Could you check a few things on this model? Use its own coordinates, in mm. Face numbers are marked on the shaded views. A direction names the side the tool comes from. Coordinates: 2 decimals unless noted, no trailing zeros. Order: outer loops, then holes, each group sorted by start corner. A loop starts at its lowest first (then second) coordinate and runs counter-clockwise, first axis right, second up. Notation, with made-up numbers: (86.5, 77) - (134.5, 77) arc R30 ccw to (134.5, 110) - close; hole circle Ø8 at (-4.5, 28). An arc over 180 degrees is marked (long way). Answer as CSV lines item,"result". Start each with the question number.
1. For the marked faces 4, 5, 6 and 7, which set-ups out of +Z, -Z, +X, -X, +Y, -Y let a thin tool reach every point of the face, with its end or its side?
2. I want a section at D-D, the plane z = -18. List the corners of the cut face in (x, y) for me, and give its area (3 significant figures).
3. I want a section at B-B, the plane y = 3. List the corners of the cut face in (x, z) for me, and give its area (3 significant figures).
4. I want a section at A-A, the plane z = 0. List the corners of the cut face in (x, y) for me.
5. I need wall thicknesses on probe 1 along X at (y, z) = (3.65, 0); probe 2 along Z at (x, y) = (15.75, 3); probe 3 along Z at (x, y) = (-1.75, 2.25). Which ranges of each line are inside material? Lowest first, please.
6. For pin 1 (1.2 mm diameter, centred on x = 8, y = 8.5, fed in from +Z); pin 2 (6 mm diameter, centred on y = 7.5, z = -29.5, fed in from +X); pin 3 (0.9 mm diameter, centred on x = 7.5, y = 2.5, fed in from +Z); pin 4 (3 mm diameter, centred on x = 0, z = 0, fed in from +Y), each with a flat end and sliding along its axis, tell me the tip position at first contact or that it passes through.
7. I want a section at C-C, the plane x = 15. List the corners of the cut face in (y, z) for me, and give its area (3 significant figures).
8. Thinking about a two-plate mould opening in X: for the marked faces 1, 2 and 3, which applies, released by +X, released by -X, zero draft, split by the parting line, or undercut?
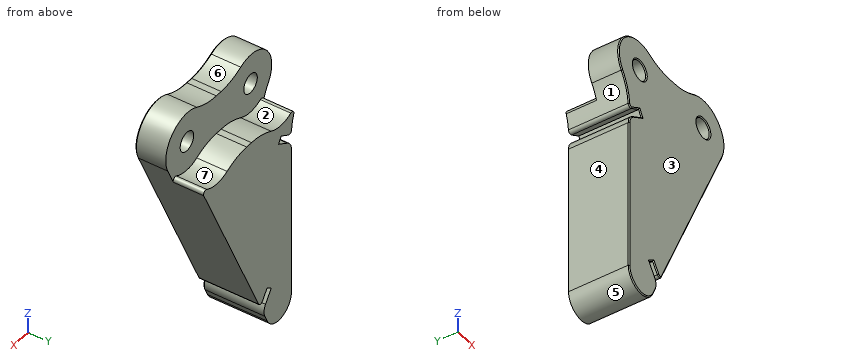
from build123d import *

# Parameters (mm, degrees)
MAIN_BODY_DEPTH                           = 10
SKETCH1_3_R                               = 1.6
CONNECTOR_BODY_DEPTH                      = 5
DULLING_FILLET_START                      = 5
DULLING_FILLET_DEPTH                      = 6
CUT_EXTRUDE1_DEPTH                        = 45.806187552
FILLET1_R                                 = 2
FILLET2_R                                 = 0.5
ELEPHANTSFOOT_COMPENSATION_LEFT_CONF_SIZE = 0.16


with BuildPart() as part:
    # complete_sketch → main_body (new body)
    with BuildSketch(Plane(origin=(0, 0, 0), x_dir=(1, 0, 0), z_dir=(0, 1, 0))):
        with BuildLine():
            ThreePointArc((-2.5, 8.291561976), (-2.925728922, 5.40481063), (-4.166666667, 2.763853992))
            ThreePointArc((-4.166666667, 2.763853992), (-1.24767584, 4.841828683), (2.312045751, 4.433333333))
            ThreePointArc((2.312045751, 4.433333333), (4.555661111, 3.587465144), (6.936137254, 3.3))
            Line((6.936137254, 3.3), (8.063862746, 3.3))
            ThreePointArc((8.063862746, 3.3), (10.444338889, 3.587465144), (12.687954249, 4.433333333))
            ThreePointArc((12.687954249, 4.433333333), (16.605433979, 4.735248857), (19.531538935, 2.113091309))
            Line((19.531538935, 2.113091309), (3.218923361, 37.095608299))
            ThreePointArc((3.218923361, 37.095608299), (-0.149318842, 38.756641535), (-2.5, 35.827753514))
            Line((-2.5, 35.827753514), (-2.5, 8.291561976))
        make_face()
    extrude(amount=MAIN_BODY_DEPTH)

    # Sketch1<3> → connector_body (add)
    with BuildSketch(Plane(origin=(0, 0, 0), x_dir=(1, 0, 0), z_dir=(0, 1, 0))):
        with BuildLine():
            ThreePointArc((2.312045751, -4.433333333), (4.555661111, -3.587465144), (6.936137254, -3.3))
            Line((6.936137254, -3.3), (8.063862746, -3.3))
            ThreePointArc((8.063862746, -3.3), (10.444338889, -3.587465144), (12.687954249, -4.433333333))
            ThreePointArc((12.687954249, -4.433333333), (18.456219958, -3.613107195), (19.531538935, 2.113091309))
            ThreePointArc((19.531538935, 2.113091309), (16.605433979, 4.735248857), (12.687954249, 4.433333333))
            ThreePointArc((12.687954249, 4.433333333), (10.444338889, 3.587465144), (8.063862746, 3.3))
            Line((8.063862746, 3.3), (6.936137254, 3.3))
            ThreePointArc((6.936137254, 3.3), (4.555661111, 3.587465144), (2.312045751, 4.433333333))
            ThreePointArc((2.312045751, 4.433333333), (-1.24767584, 4.841828683), (-4.166666667, 2.763853992))
            ThreePointArc((-4.166666667, 2.763853992), (-3.716151374, -3.345178466), (2.312045751, -4.433333333))
        make_face()
        with Locations(Location((0, 0, 0), (0, 0, 270))):
            Circle(SKETCH1_3_R, mode=Mode.SUBTRACT)
        with Locations(Location((15, 0, 0), (0, 0, 270))):
            Circle(SKETCH1_3_R, mode=Mode.SUBTRACT)
    extrude(amount=CONNECTOR_BODY_DEPTH)

    # dulling_fillet: read off the stored shape, not the designer's step
    # dulling_fillet outline → dulling_fillet (cut)
    with BuildSketch(Plane(origin=(0, 0, 0), x_dir=(1, 0, 0), z_dir=(0, 1, 0)).offset(DULLING_FILLET_START)):
        with BuildLine():
            Line((19.531538935, 2.113091309), (18.195102647, 4.979088177))
            ThreePointArc((18.195102647, 4.979088177), (18.080055144, 4.399425861), (17.492680685, 4.334344587))
            ThreePointArc((17.492680685, 4.334344587), (18.683531845, 3.381063908), (19.531538935, 2.113091309))
        make_face()
        with BuildLine():
            ThreePointArc((-4.166666667, 2.763853992), (-3.358016887, 3.704554303), (-2.342670216, 4.417227214))
            ThreePointArc((-2.342670216, 4.417227214), (-2.902133749, 4.479151002), (-3.049464036, 5.022407651))
            ThreePointArc((-3.049464036, 5.022407651), (-3.536643042, 3.85780149), (-4.166666667, 2.763853992))
        make_face()
    extrude(amount=DULLING_FILLET_DEPTH, mode=Mode.SUBTRACT)

    # Sketch2 → Cut-Extrude1 (cut, through all)
    with BuildSketch(Plane(origin=(0, 10, 0), x_dir=(1, 0, 0), z_dir=(0, 1, 0))):
        Polygon((-2.5, 8.291561976), (-0.068911087, 6.887972137), (0.531088913, 7.927202622), (-2.5, 9.677202622), align=None)
        Polygon((4.275469015, 34.829838831), (2.267951488, 31.962806676), (3.250933941, 31.274514953), (4.861066057, 33.574021924), align=None)
    extrude(amount=-CUT_EXTRUDE1_DEPTH, mode=Mode.SUBTRACT)

    # Fillet1
    fillet1_edges = [part.edges().sort_by_distance(p)[0] for p in [
        (-2.5, 5, -9.677202622),
        (4.275469015, 5, -34.829838831),
    ]]
    fillet(fillet1_edges, radius=FILLET1_R)

    # Fillet2
    fillet2_edges = [part.edges().sort_by_distance(p)[0] for p in [
        (4.861066057, 5, -33.574021924),
        (-2.5, 5, -8.291561976),
    ]]
    fillet(fillet2_edges, radius=FILLET2_R)

    # elephantsfoot_compensation_left_conf
    elephantsfoot_compensation_left_conf_edges = [part.edges().sort_by_distance(p)[0] for p in [
        (0.231088913, 0, -7.40758738),
        (3.807634117, 0, -32.069565198),
        (2.759442715, 0, -31.618660815),
        (-2.5, 0, -23.329828337),
        (2.940555742, 0, -32.923385101),
        (-0.149318842, 0, -38.756641535),
        (3.503197421, 0, -36.48598061),
        (-2.232050808, 0, -9.83190316),
        (3.967245303, 0, -34.856804912),
        (12.379301571, 0, -17.451113833),
        (-3.049950658, 0, -5.021001256),
        (-0.926536362, 0, -7.383122321),
        (-2.266493544, 0, -7.888003391),
        (4.817488185, 0, -33.075924575),
        (-3.716151374, 0, 3.345178466),
        (18.456219958, 0, 3.613107195),
        (7.5, 0, 3.3),
        (10.444338889, 0, 3.587465144),
        (0, 0, -1.6),
        (15, 0, -1.6),
        (4.555661111, 0, 3.587465144),
        (-0.484455543, 0, -8.513527487),
    ]]
    chamfer(elephantsfoot_compensation_left_conf_edges, length=ELEPHANTSFOOT_COMPENSATION_LEFT_CONF_SIZE)


solid = part.part
Solved:
1,face 4,"-Z, -X, +Y, -Y"
1,face 5,"-Z, +Y, -Y"
1,face 6,"+Z, +Y, -Y"
1,face 7,"+Z, +Y"
2,outline,"(-2.5, 0.16) - (-2.34, 0) - (11.95, 0) - (12.12, 0.16) - (12.12, 10) - (-2.5, 10) - close"
2,area,"146 mm2"
3,outline,"(-4.17, -2.76) arc R10 cw to (-2.53, -7.49) arc R0.5 ccw to (-1.78, -7.88) - (-0.07, -6.89) - (0.53, -7.93) - (-1.5, -9.1) arc R2 ccw to (-2.5, -10.83) - (-2.5, -35.83) arc R3 ccw to (3.22, -37.1) - (3.79, -35.88) arc R2 ccw to (3.61, -33.88) - (2.27, -31.96) - (3.25, -31.27) - (4.36, -32.86) arc R0.5 ccw to (5.23, -32.79) - (19.53, -2.11) arc R5 ccw to (12.69, 4.43) arc R10 cw to (8.06, 3.3) - (6.94, 3.3) arc R10 cw to (2.31, 4.43) arc R5 ccw to start; hole circle Ø3.2 at (0, 0); hole circle Ø3.2 at (15, 0)"
3,area,"623 mm2"
4,outline,"(-5, 0.16) - (-4.84, 0) - (-1.76, 0) - (-1.6, 0.16) - (-1.6, 5) - (-5, 5) - close; (1.6, 0.16) - (1.76, 0) - (13.24, 0) - (13.4, 0.16) - (13.4, 5) - (1.6, 5) - close; (16.6, 0.16) - (16.76, 0) - (19.84, 0) - (20, 0.16) - (20, 5) - (16.6, 5) - close"
5,probe 1,"x = -5 to -1.6, 1.6 to 13.4, 16.6 to 20"
5,probe 2,"z = -10.22 to -1.41, 1.41 to 4.94"
5,probe 3,"z = -37.81 to -9.27, -7.86 to 4.68"
6,pin 1,"stops at z = -3.3"
6,pin 2,"stops at x = 8.16"
6,pin 3,"stops at z = 3.3"
6,pin 4,"passes through"
7,outline,"(0, -11.45) - (0.16, -11.83) - (10, -11.83) - (10, -5) - (5, -5) - (5, -1.6) - (0.16, -1.6) - (0, -1.76) - close; (0, 1.76) - (0.16, 1.6) - (5, 1.6) - (5, 5) - (0.16, 5) - (0, 4.84) - close"
7,area,"102 mm2"
8,face 1,"released by -X"
8,face 2,"undercut"
8,face 3,"zero draft"
